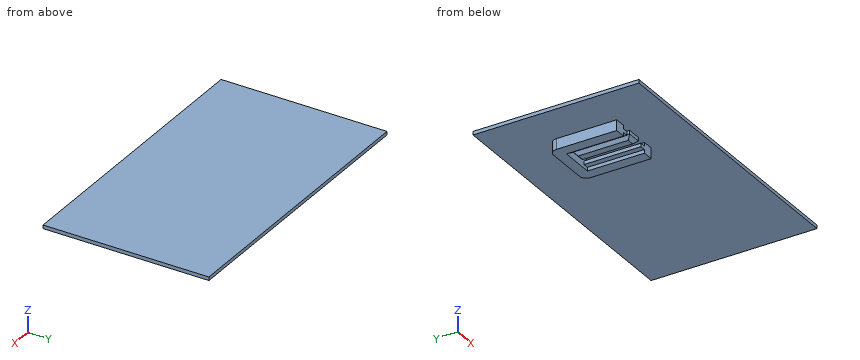
from build123d import *

# Parameters (mm, degrees)
F2_DEPTH = 2.5
F3_DEPTH = 2.5
F4_DEPTH = 2.5
F4_TAPER = 45
F5_W     = 7.8047607094
F5_H     = 40.5
F5_H_2   = 7.430572629
F5_W_2   = 7.7738855034
F6_DEPTH = 2.5
F7_R     = 5
F8_W     = 204.3793946505
F8_H     = 117.8380995989
F9_DEPTH = 2.5


with BuildPart() as f2:
    # F1 (on Top) → F2 (new body)
    with BuildSketch(Plane.XY):
        Polygon((-12, 12.7071067812), (-12, 16), (-12, 20.5), (-8, 20.5), (-5, 20.5), (5, 20.5), (8, 20.5), (12, 20.5), (12, -20), (19.7742227465, -20), (19.7742227465, 27.930572629), (-19.7742227465, 27.930572629), (-19.7742227465, -20), (-12, -20), align=None)
        Polygon((5, 20.5), (-5, 20.5), (-5, -20), (5, -20), (5, 12.7071067812), (5, 16), align=None)
    extrude(amount=F2_DEPTH)

    # F1 (on Top) → F3 (join)
    with BuildSketch(Plane.XY):
        Polygon((12, 20.5), (8, 20.5), (8, 16), (8.2928932188, 16), (8, 15.7071067812), (8, -20), (12, -20), align=None)
        Polygon((-12, 12.7071067812), (-12, 16), (-12, 20.5), (-8, 20.5), (-5, 20.5), (5, 20.5), (8, 20.5), (12, 20.5), (12, -20), (19.7742227465, -20), (19.7742227465, 27.930572629), (-19.7742227465, 27.930572629), (-19.7742227465, -20), (-12, -20), align=None)
        Polygon((8.2928932188, 16), (8, 16), (8, 15.7071067812), align=None)
        Polygon((-12, 20.5), (-12, 16), (-8.7071067812, 16), (-12, 12.7071067812), (-12, -20), (-8, -20), (-8, 20.5), align=None)
        Polygon((-8.7071067812, 16), (-12, 16), (-12, 12.7071067812), align=None)
    extrude(amount=-F3_DEPTH)

    # F1 (on Top) → F4 (join)
    with BuildSketch(Plane.XY):
        Polygon((5, 20.5), (-5, 20.5), (-5, -20), (5, -20), (5, 12.7071067812), (5, 16), align=None)
    extrude(amount=-F4_DEPTH, taper=F4_TAPER)

    # F5 (on face) → F6 (join)
    with BuildSketch(Plane(origin=(0, 0, -2.5), x_dir=(1, 0, 0), z_dir=(0, 0, -1))):
        with Locations((-15.8718423918, -0.25)):
            Rectangle(F5_W, F5_H)
        with Locations((-15.8718423918, -24.2152863145)):
            Rectangle(F5_W, F5_H_2)
        with Locations((15.8872799948, -0.25)):
            Rectangle(F5_W_2, F5_H)
        with Locations((15.8872799948, -24.2152863145)):
            Rectangle(F5_W_2, F5_H_2)
        Polygon((-8, -20.5), (-11.9694620371, -20.5), (-11.9694620371, -27.930572629), (12.0003372431, -27.930572629), (12.0003372431, -20.5), (8, -20.5), align=None)
    extrude(amount=F6_DEPTH)

    # F7
    f7_edges = [f2.edges().sort_by_distance(p)[0] for p in [
        (-19.774223, 27.930573, -1.25),
        (19.774223, 27.930573, -1.25),
    ]]
    fillet(f7_edges, radius=F7_R)

    # F8 (on face) → F9 (join)
    with BuildSketch(Plane.XY.offset(2.5)):
        with Locations((52.1517619491, 4.441536963)):
            Rectangle(F8_W, F8_H)
        with BuildLine():
            Line((19.7742227465, 22.930572629), (19.7742227465, -20))
            Line((19.7742227465, -20), (12, -20))
            Line((12, -20), (12, 20.5))
            Line((12, 20.5), (5, 20.5))
            Line((5, 20.5), (5, -20))
            Line((5, -20), (-5, -20))
            Line((-5, -20), (-5, 20.5))
            Line((-5, 20.5), (-12, 20.5))
            Line((-12, 20.5), (-12, -20))
            Line((-12, -20), (-19.7742227465, -20))
            Line((-19.7742227465, -20), (-19.7742227465, 22.930572629))
            ThreePointArc((-19.7742227465, 22.930572629), (-18.3097566524, 26.4661065349), (-14.7742227465, 27.930572629))
            Line((-14.7742227465, 27.930572629), (14.7742227465, 27.930572629))
            ThreePointArc((14.7742227465, 27.930572629), (18.3097566524, 26.4661065349), (19.7742227465, 22.930572629))
        make_face(mode=Mode.SUBTRACT)
        with BuildLine():
            Line((12, -20), (19.7742227465, -20))
            Line((19.7742227465, -20), (19.7742227465, 22.930572629))
            ThreePointArc((19.7742227465, 22.930572629), (18.3097566524, 26.4661065349), (14.7742227465, 27.930572629))
            Line((14.7742227465, 27.930572629), (-14.7742227465, 27.930572629))
            ThreePointArc((-14.7742227465, 27.930572629), (-18.3097566524, 26.4661065349), (-19.7742227465, 22.930572629))
            Line((-19.7742227465, 22.930572629), (-19.7742227465, -20))
            Line((-19.7742227465, -20), (-12, -20))
            Line((-12, -20), (-12, 20.5))
            Line((-12, 20.5), (-5, 20.5))
            Line((-5, 20.5), (-5, -20))
            Line((-5, -20), (5, -20))
            Line((5, -20), (5, 20.5))
            Line((5, 20.5), (12, 20.5))
            Line((12, 20.5), (12, -20))
        make_face()
    extrude(amount=F9_DEPTH)


solid = f2.part
The listing builds one solid part. Answer for the finished solid, in the listing's coordinates (mm). Round coordinates to 2 decimals unless told otherwise and drop trailing zeros. Order: outer loops, then holes, each group sorted by start corner. A loop starts at its lowest first (then second) coordinate and runs counter-clockwise, first axis right, second up. Notation, with made-up numbers: (38, 32.25) - (68, 32.25) arc R16 cw to (68, 40.25) - close; hole circle Ø8 at (-3, 80.5). An arc over 180 degrees is marked (long way). Write item = value, one per line. Start each with the question number.
1) Section B-B, the plane x = 125.5 is taken. Write down the section's boundary in (y, z), plus the area to 3 significant figures.
2) Section A-A, the plane y = -42 is taken. Write down the section's boundary in (x, z), plus the area to 3 significant figures.
3) Given pin 1 (1.5 mm diameter, centred on x = 89.5, y = 41, fed in from -Z); pin 2 (3 mm diameter, centred on y = 4, z = -3.5, fed in from +X); pin 3 (3 mm diameter, centred on x = 4.5, z = -1.5, fed in from +Y); pin 4 (1.5 mm diameter, centred on x = 60.5, z = 1, fed in from -Y), each flat-ended and moving along its own axis, determine where each tip first touches the part or whether it passes through.
4) Straight lines are drawn through the part: L1, parallel to X at y = -14, z = 2; L2, parallel to X at y = -18.5, z = -4; L3, parallel to X at y = -9, z = -0.75. For each, find the intervals that lie inside material, in ascending order.
Results list:
q1.outline = (-54.48, 2.5) - (63.36, 2.5) - (63.36, 5) - (-54.48, 5) - close
q1.area = 295 mm^2
q2.outline = (-50.04, 2.5) - (154.34, 2.5) - (154.34, 5) - (-50.04, 5) - close
q2.area = 511 mm^2
q3.pin_1 = 2.5
q3.pin_2 = 19.77
q3.pin_3 = 27.93
q3.pin_4 = through
q4.L1 = -19.77 to -12, -5 to 5, 12 to 19.77
q4.L2 = -19.77 to -11.97, 12 to 19.77
q4.L3 = -19.77 to -8, -4.25 to 4.25, 8 to 19.77
